The figure shows three views and two pictorial views of one solid part (mm, origin at its lowest corner). Answer the questions. A direction names the side the tool comes from. Coordinates: 2 decimals unless noted, no trailing zeros. Loops run counter-clockwise (first coordinate to the right, second up) from the corner with the lowest first, then second, coordinate; pieces in that order, holes last. Notation, with made-up numbers: (-31, 79.5) - (5, 79.5) arc R13 ccw to (5, 98.5) - close; hole circle Ø4 at (-2.5, 40.25). An arc over 180 degrees is marked (long way). Return JSON: item names as keys, results as strings. Group by question number.
1. Section C-C (y = 48.5) is taken. Write down the section's boundary in (x, z).
2. Section D-D (x = 42) is taken. Write down the section's boundary in (y, z) (1 decimal).
3. Find the intervals of material crossed by line 1 along Z through (x, y) = (9, 34.5); line 2 along X through (y, z) = (23.5, 4.5); line 3 along X through (y, z) = (53, 0.5), in increasing order.
4. Which of the six approach directions +Z, -Z, +X, -X, +Y, -Y give full straight-line access (tool end or side, diameter ignored) to the marked faces 4, 5, 6 and 7?
5. The mould has two halves that part along Y. Classify the marked faces 1, 2 and 3: pulls with the +Y half, pulls with the -Y half, needs draft (parallel to the pull), parting line crosses it, or undercut.
6. Each of these flat-tipped pins is pushed along its axis until it touches: P1, Ø1, axis at x = 9, z = 3, coming from the +Y side; P2, Ø6, axis at x = 19.5, z = 9.5, coming from the -Y side. Where does it stop, or does it pass through?
7. Section A-A (x = 7) is taken. Write down the section's boundary in (y, z).
8. Section B-B (z = 8.75) is taken. Write down the section's boundary in (x, y) (1 decimal).
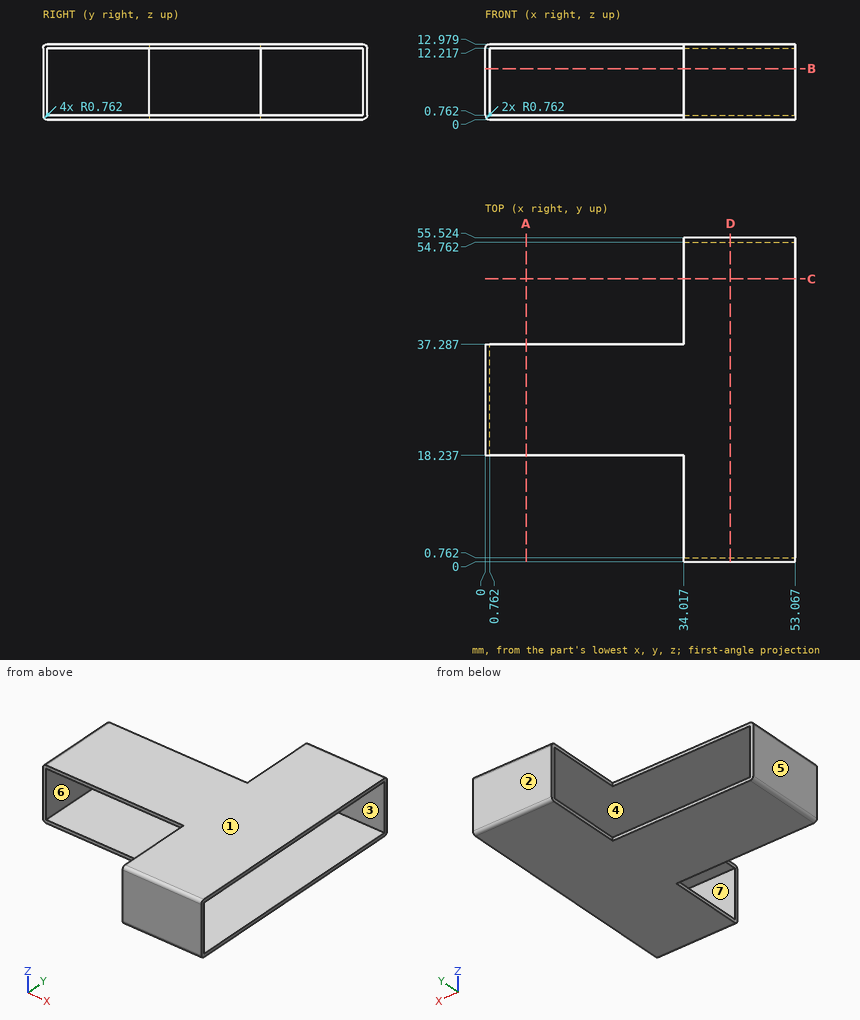
The answers:
{
 "1": {"outline": "(34.02, 0) - (53.07, 0) - (53.07, 0.76) - (34.02, 0.76) - close; (34.02, 12.22) - (53.07, 12.22) - (53.07, 12.98) - (34.02, 12.98) - close"},
 "2": {"outline": "(0, 0.8) arc R0.8 ccw to (0.8, 0) - (54.8, 0) arc R0.8 ccw to (55.5, 0.8) - (55.5, 12.2) arc R0.8 ccw to (54.8, 13) - (0.8, 13) arc R0.8 ccw to (0, 12.2) - close; hole (0.8, 0.8) - (54.8, 0.8) - (54.8, 12.2) - (0.8, 12.2) - close"},
 "3": {"line 1": "z = 0 to 0.76, 12.22 to 12.98", "line 2": "x = 0 to 0.76", "line 3": "x = 34.02 to 53.07"},
 "4": {"face 4": "+X", "face 5": "+Z, -Z, -X, +Y, -Y", "face 6": "+X, +Y, -Y", "face 7": "+X, -X"},
 "5": {"face 1": "needs draft", "face 2": "pulls with the +Y half", "face 3": "undercut"},
 "6": {"P1": "passes through", "P2": "stops at y = 18.24"},
 "7": {"outline": "(18.24, 0) - (37.29, 0) - (37.29, 0.76) - (18.24, 0.76) - close; (18.24, 12.22) - (37.29, 12.22) - (37.29, 12.98) - (18.24, 12.98) - close"},
 "8": {"outline": "(0, 18.2) - (0.8, 18.2) - (0.8, 37.3) - (0, 37.3) - close; (34, 0) - (53.1, 0) - (53.1, 0.8) - (34, 0.8) - close; (34, 54.8) - (53.1, 54.8) - (53.1, 55.5) - (34, 55.5) - close"}
}
